Could you check a few things on this model? Use its own coordinates, in mm. Give positions to 0.01 mm unless a question says otherwise; leave off trailing zeros. Loops run counter-clockwise (first coordinate to the right, second up) from the corner with the lowest first, then second, coordinate; pieces in that order, holes last. Notation, with made-up numbers: M -22.75,84.5 L 3.25,84.5 A9 cw 3.25,93.5 Z; hole C 40,80.5 d9. An arc over 180 degrees is marked long. Use a Markdown table: item, result. Add a question column.
1) Suppose I cut it at A-A on z = 0. List the corners of the cut face in (x, y) for me.
2) Suppose I cut it at C-C on x = 0. List the corners of the cut face in (y, z) for me.
3) Suppose I cut it at B-B on y = 1.9. List the corners of the cut face in (x, z) for me.
4) If I drill on line 1 along X through (y, z) = (2.2, 0); line 2 along Z through (x, y) = (1.25, 2.35), over which ranges is the centre line in solid material (lowest first)? Write a range as [from, to].
5) We'd pull the mould along X, two halves only. Please class faces 1 (the flat face through (3.45, 2, 0)), 2 (the cylindrical face through (-0.5, 2.5, 2.4)), 3 (the flat face through (-2.227, 2.465, 2.208)), 4 (the flat face through (0, 2, 3.45)): +X half, -X half, draft (parallel to the pull), parting line (faces both ways), or undercut.
6) Will this pin go through, and if not, where does the flat tip stop? pin 1 Ø1 at (y, z) = (1.5, 2.5) entering from +X.
7) Suppose I cut it at D-D on z = 2.75. List the corners of the cut face in (x, y) for me, and give its area (3 significant figures).
```python
from build123d import *

# Parameters (mm, degrees)
CROQUIS1_R              = 2.45
SALIENTE_EXTRUIR1_DEPTH = 5


with BuildPart() as part:
    # Croquis1 → Saliente-Extruir1 (new body)
    with BuildSketch(Plane(origin=(0, 0, 0), x_dir=(1, 0, 0), z_dir=(0, 1, 0))):
        Polygon((0.029803377, 3.449555781), (-0.970196623, 3.449555781), (-3.45, 1), (-3.45, -1), (-0.970196623, -3.449555781), (0.029803377, -3.449555781), (1.029803377, -3.449555781), (3.45, -1), (3.45, 1), (1.029803377, 3.449555781), align=None)
        Circle(CROQUIS1_R, mode=Mode.SUBTRACT)
    extrude(amount=SALIENTE_EXTRUIR1_DEPTH)


solid = part.part
```
Answer block:
| question | item | result |
|---|---|---|
| 1 | outline | M -3.45,0 L -2.45,0 L -2.45,5 L -3.45,5 Z; M 2.45,0 L 3.45,0 L 3.45,5 L 2.45,5 Z |
| 2 | outline | M 0,-3.45 L 5,-3.45 L 5,-2.45 L 0,-2.45 Z; M 0,2.45 L 5,2.45 L 5,3.45 L 0,3.45 Z |
| 3 | outline | M -3.45,-1 L -0.97,-3.45 L 1.03,-3.45 L 3.45,-1 L 3.45,1 L 1.03,3.45 L -0.97,3.45 L -3.45,1 Z; hole C 0,0 d4.9 |
| 4 | line 1 | x = [-3.45, -2.45], [2.45, 3.45] |
| 4 | line 2 | z = [-3.23, -2.11], [2.11, 3.23] |
| 5 | face 1 | +X half |
| 5 | face 2 | undercut |
| 5 | face 3 | -X half |
| 5 | face 4 | draft |
| 6 | pin 1 | stops at x = 2.46 |
| 7 | outline | M -1.68,0 L 1.72,0 L 1.72,5 L -1.68,5 Z |
| 7 | area | 17.0 mm^2 |
